from build123d import *

# Parameters (mm, degrees)
ESQUISSE1_W             = 20
ESQUISSE1_H             = 78
BOSS_EXTRU_1_DEPTH      = 33
ESQUISSE2_W             = 20
ESQUISSE2_H             = 8
BOSS_EXTRU_2_DEPTH      = 20
ESQUISSE3_W             = 20
ESQUISSE3_H             = 8
BOSS_EXTRU_3_DEPTH      = 20
ESQUISSE4_R             = 4
ENL_V_MAT_EXTRU_1_DEPTH = 10
CONG_1_R                = 5
ESQUISSE5_R             = 28.5
ENL_V_MAT_EXTRU_2_DEPTH = 30
ESQUISSE6_R             = 2.6
ENL_V_MAT_EXTRU_3_DEPTH = 20
CONG_4_R                = 15
CONG_5_R                = 3
ESQUISSE7_R             = 29.5
ENL_V_MAT_EXTRU_4_DEPTH = 4


with BuildPart() as part:
    # Esquisse1 → Boss.-Extru.1 (new body)
    with BuildSketch(Plane.XY):
        with Locations((10, 39)):
            Rectangle(ESQUISSE1_W, ESQUISSE1_H)
    extrude(amount=BOSS_EXTRU_1_DEPTH)

    # Esquisse2 → Boss.-Extru.2 (add)
    with BuildSketch(Plane(origin=(0, 78, 0), x_dir=(1, 0, 0), z_dir=(0, 1, 0))):
        with Locations((10, -4)):
            Rectangle(ESQUISSE2_W, ESQUISSE2_H)
    extrude(amount=BOSS_EXTRU_2_DEPTH)

    # Esquisse3 → Boss.-Extru.3 (add)
    with BuildSketch(Plane.XZ):
        with Locations((10, 4)):
            Rectangle(ESQUISSE3_W, ESQUISSE3_H)
    extrude(amount=BOSS_EXTRU_3_DEPTH)

    # Esquisse4 → Enlèv. mat.-Extru.1 (cut)
    with BuildSketch(Plane.XY.offset(8)):
        with Locations((10, 87)):
            Circle(ESQUISSE4_R)
        with Locations(Location((10, -9, 0), (0, 0, 180))):
            Circle(ESQUISSE4_R)
    extrude(amount=-ENL_V_MAT_EXTRU_1_DEPTH, mode=Mode.SUBTRACT)

    # Congé1
    cong_1_edges = [part.edges().sort_by_distance(p)[0] for p in [
        (0, 98, 4),
        (20, 98, 4),
        (0, -20, 4),
        (20, -20, 4),
    ]]
    fillet(cong_1_edges, radius=CONG_1_R)

    # Esquisse5 → Enlèv. mat.-Extru.2 (cut)
    with BuildSketch(Plane(origin=(20, 0, 0), x_dir=(0, 0, -1), z_dir=(1, 0, 0))):
        with Locations((0, 39)):
            Circle(ESQUISSE5_R)
    extrude(amount=-ENL_V_MAT_EXTRU_2_DEPTH, mode=Mode.SUBTRACT)

    # Esquisse6 → Enlèv. mat.-Extru.3 (cut)
    with BuildSketch(Plane(origin=(20, 0, 0), x_dir=(0, 0, -1), z_dir=(1, 0, 0))):
        with Locations((-23.528978144, 15.471021856)):
            Circle(ESQUISSE6_R)
        with Locations((-23.528978144, 62.528978144)):
            Circle(ESQUISSE6_R)
    extrude(amount=-ENL_V_MAT_EXTRU_3_DEPTH, mode=Mode.SUBTRACT)

    # Congé4
    cong_4_edges = [part.edges().sort_by_distance(p)[0] for p in [
        (10, 78, 33),
        (10, 0, 33),
    ]]
    fillet(cong_4_edges, radius=CONG_4_R)

    # Congé5
    cong_5_edges = [part.edges().sort_by_distance(p)[0] for p in [
        (0, 39, 33),
        (20, 39, 33),
        (20, 78, 13),
        (20, 0, 13),
        (20, 73.606601718, 28.606601718),
        (20, 4.393398282, 28.606601718),
        (0, 0, 13),
        (0, 78, 13),
        (0, 73.606601718, 28.606601718),
        (0, 4.393398282, 28.606601718),
    ]]
    fillet(cong_5_edges, radius=CONG_5_R)

    # Esquisse7 → Enlèv. mat.-Extru.4 (cut)
    with BuildSketch(Plane.ZY):
        with Locations((0, 39)):
            Circle(ESQUISSE7_R)
    extrude(amount=-ENL_V_MAT_EXTRU_4_DEPTH, mode=Mode.SUBTRACT)


solid = part.part
Build history of the part. All positions in model axes, mm. A direction names the side the tool comes from. Coordinates: 2 decimals unless noted, no trailing zeros. Write each loop counter-clockwise with the first axis right and the second up, starting at its lowest first coordinate (ties: lowest second). Pieces come first, ordered by that corner, then holes.
(1) Drill centre lines: line 1 (Y direction, x = 18, z = 22.5); line 2 (X direction, y = -9, z = 5); line 3 (Z direction, x = 10.5, y = 39.5). Where is each one in solid material? Low to high.
(2) Mould opens along Z. For faces 4 (the cylindrical face through (12.112, 39.627, 28.493)), 5 (the cylindrical face through (10.14, 14.475, 21.127)), 6 (the flat face through (0, 43.3, 29.4)) say: pulls with the +Z half, pulls with the -Z half, needs draft (parallel to the pull), parting line crosses it, or undercut.
(3) Cut at A-A on x = 11.25. List the corners of the cut face in (y, z), and give its area (3 significant figures).
(4) Cut at D-D on z = 15.5. List the corners of the cut face in (x, y), and give its area (3 significant figures).
(5) 3-axis set-ups, long thin cutter, end or side, ignore diameter. For faces 1 (the flat face through (10, 0, 13)), 2 (the cylindrical face through (1.972, 38.351, 29.493)), 3 (the flat face through (10, 78, 13)): which of +Z, -Z, +X, -X, +Y, -Y reach the whole face in a straight line?
(6) Pin check, flat tips, straight feed: pin 1 Ø10 at (x, y) = (11.5, 86.5) entering from +Z; pin 2 Ø9 at (x, y) = (10, -9) entering from -Z; pin 3 Ø4 at (x, z) = (18, 6.5) entering from -Y; pin 4 Ø2 at (y, z) = (77, 10) entering from -X. Stop position of each tip, or through.
(7) Cut at B-B on y = -9. List the corners of the cut face in (x, z).
(8) Cut at C-C on y = 39. List the corners of the cut face in (x, z), and give its area (3 significant figures).
Working result:
1. line 1: y = 0.87 to 13.08, 17.86 to 21.51, 56.49 to 60.14, 64.92 to 77.13
1. line 2: x = 0 to 6, 14 to 20
1. line 3: z = 28.5 to 33
2. face 4: pulls with the -Z half
2. face 5: undercut
2. face 6: needs draft
3. outline: (-20, 0) - (-12.8, 0) - (-12.8, 8) - (-20, 8) - close; (-5.2, 0) - (10.5, 0) arc R28.5 cw to (67.5, 0) - (83.2, 0) - (83.2, 8) - (78, 8) - (78, 18) arc R15 ccw to (63, 33) - (15, 33) arc R15 ccw to (0, 18) - (0, 8) - (-5.2, 8) - close; (90.8, 0) - (98, 0) - (98, 8) - (90.8, 8) - close; hole circle Ø5.2 at (15.47, 23.53); hole circle Ø5.2 at (62.53, 23.53)
3. area: 1,360 mm2
4. outline: (0, 3) arc R3 ccw to (3, 0) - (17, 0) arc R3 ccw to (20, 3) - (20, 15.08) - (4, 15.08) - (4, 13.9) - (0, 13.9) - close; (0, 64.1) - (4, 64.1) - (4, 62.92) - (20, 62.92) - (20, 75) arc R3 ccw to (17, 78) - (3, 78) arc R3 ccw to (0, 75) - close
4. area: 586 mm2
5. face 1: +Z, +X, -X, -Y
5. face 2: -Z, -X
5. face 3: +Z, +X, -X, +Y
6. pin 1: stops at z = 8
6. pin 2: stops at z = 0
6. pin 3: stops at y = -19.9
6. pin 4: stops at x = 0.17
7. outline: (0, 0) - (6, 0) - (6, 8) - (0, 8) - close; (14, 0) - (20, 0) - (20, 8) - (14, 8) - close
8. outline: (0, 29.5) - (4, 29.5) - (4, 28.5) - (20, 28.5) - (20, 30) arc R3 ccw to (17, 33) - (3, 33) arc R3 ccw to (0, 30) - close
8. area: 82.1 mm2
